Input: part model. Units: mm. Frame: model coordinates. Face numbers are marked on the shaded views. A direction names the side the tool comes from. Give positions to 0.01 mm unless a question says otherwise; leave off trailing zeros. Order: outer loops, then holes, each group sorted by start corner. A loop starts at its lowest first (then second) coordinate and runs counter-clockwise, first axis right, second up. Notation, with made-up numbers: M 17.25,6.5 L 57.25,6.5 A24 ccw 57.25,18.5 Z; hole C -9.75,64.5 d1. An arc over 180 degrees is marked long. Use a Markdown table: item, result.
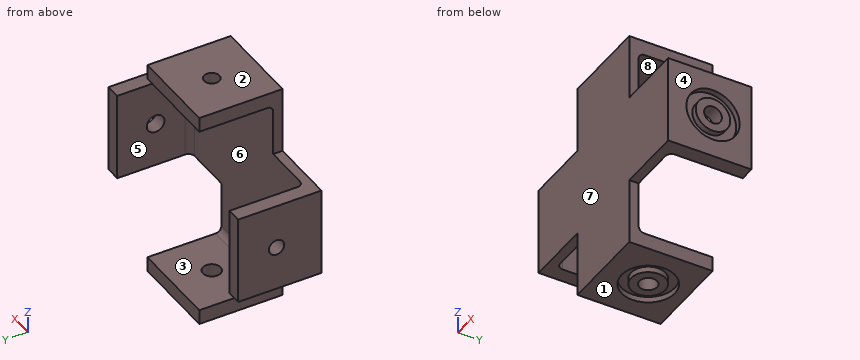
from build123d import *

# Parameters (mm, degrees)
BOSS_EXTRUDE1_DEPTH = 3.175
SKETCH4_W           = 5
SKETCH4_H           = 30
BOSS_EXTRUDE3_DEPTH = 25
FILLET1_R           = 2
SKETCH5_W           = 30
SKETCH5_H           = 5
BOSS_EXTRUDE4_DEPTH = 25
FILLET2_R           = 2
SKETCH6_R           = 2.6
CUT_EXTRUDE1_DEPTH  = 10
CIRPATTERN1_COUNT   = 2
CIRPATTERN1_ANGLE   = 90
SKETCH7_R           = 3
CUT_EXTRUDE2_DEPTH  = 10
CIRPATTERN2_COUNT   = 2
CIRPATTERN2_ANGLE   = 90
SKETCH10_R          = 9
SKETCH10_R_2        = 5.83
CUT_EXTRUDE9_DEPTH  = 2
CIRPATTERN4_COUNT   = 2
CIRPATTERN4_ANGLE   = 270


with BuildPart() as part:
    # Sketch1 → Boss-Extrude1 (new body)
    with BuildSketch(Plane(origin=(0, 0, 0), x_dir=(1, 0, 0), z_dir=(0, 1, 0))):
        Polygon((-15, 15), (-15, 37.5), (15, 37.5), (15, 15), (37.5, 15), (37.5, -15), (15, -15), (15, -37.5), (-15, -37.5), (-15, -15), (-37.5, -15), (-37.5, 15), align=None)
    extrude(amount=BOSS_EXTRUDE1_DEPTH)

    # Sketch4 → Boss-Extrude3 (add)
    with BuildSketch(Plane(origin=(0, 3.175, 0), x_dir=(1, 0, 0), z_dir=(0, 1, 0))):
        with Locations((-35, 0)):
            Rectangle(SKETCH4_W, SKETCH4_H)
        with Locations((35, 0)):
            Rectangle(SKETCH4_W, SKETCH4_H)
    extrude(amount=BOSS_EXTRUDE3_DEPTH)

    # Fillet1
    fillet1_edges = [part.edges().sort_by_distance(p)[0] for p in [
        (-32.5, 3.175, 0),
        (32.5, 3.175, 0),
    ]]
    fillet(fillet1_edges, radius=FILLET1_R)

    # Sketch5 → Boss-Extrude4 (add)
    with BuildSketch(Plane(origin=(0, 3.175, 0), x_dir=(1, 0, 0), z_dir=(0, 1, 0))):
        with Locations((0, -35)):
            Rectangle(SKETCH5_W, SKETCH5_H)
        with Locations((0, 35)):
            Rectangle(SKETCH5_W, SKETCH5_H)
    extrude(amount=BOSS_EXTRUDE4_DEPTH)

    # Fillet2
    fillet2_edges = [part.edges().sort_by_distance(p)[0] for p in [
        (0, 3.175, 32.5),
        (0, 3.175, -32.5),
    ]]
    fillet(fillet2_edges, radius=FILLET2_R)

    # Sketch6 → Cut-Extrude1 (cut)
    with BuildSketch(Plane.ZY.offset(37.5)):
        with Locations((0, 15.175)):
            Circle(SKETCH6_R)
    cut_extrude1 = extrude(amount=-CUT_EXTRUDE1_DEPTH, mode=Mode.SUBTRACT)

    # CirPattern1: Cut-Extrude1 ×2 about axis
    cirpattern1_axis = Axis((0, 3.175, 0), (0, 1, 0))
    for i in range(1, CIRPATTERN1_COUNT):
        add(cut_extrude1.rotate(cirpattern1_axis, i * CIRPATTERN1_ANGLE / (CIRPATTERN1_COUNT - 1)), mode=Mode.SUBTRACT)

    # Sketch7 → Cut-Extrude2 (cut)
    with BuildSketch(Plane(origin=(37.5, 0, 0), x_dir=(0, 0, -1), z_dir=(1, 0, 0))):
        with Locations((0, 15.175)):
            Circle(SKETCH7_R)
    cut_extrude2 = extrude(amount=-CUT_EXTRUDE2_DEPTH, mode=Mode.SUBTRACT)

    # CirPattern2: Cut-Extrude2 ×2 about axis
    cirpattern2_axis = Axis((0, 3.175, 0), (0, 1, 0))
    for i in range(1, CIRPATTERN2_COUNT):
        add(cut_extrude2.rotate(cirpattern2_axis, i * CIRPATTERN2_ANGLE / (CIRPATTERN2_COUNT - 1)), mode=Mode.SUBTRACT)

    # Sketch10 → Cut-Extrude9 (cut)
    with BuildSketch(Plane(origin=(0, 0, -37.5), x_dir=(-1, 0, 0), z_dir=(0, 0, -1))):
        with Locations((0, 15.175)):
            Circle(SKETCH10_R)
        with Locations((0, 15.175)):
            Circle(SKETCH10_R_2, mode=Mode.SUBTRACT)
    cut_extrude9 = extrude(amount=-CUT_EXTRUDE9_DEPTH, mode=Mode.SUBTRACT)

    # CirPattern4: Cut-Extrude9 ×2 about axis
    cirpattern4_axis = Axis((0, 3.175, 0), (0, 1, 0))
    for i in range(1, CIRPATTERN4_COUNT):
        add(cut_extrude9.rotate(cirpattern4_axis, i * CIRPATTERN4_ANGLE / (CIRPATTERN4_COUNT - 1)), mode=Mode.SUBTRACT)


solid = part.part
1) Reachability of the marked faces 4, 5, 6, 7 and 8 from +Z, -Z, +X, -X, +Y, -Y: full face, straight path, thin tool, end or side. Return the list, or none.
Response values:
| item | result |
|---|---|
| face 4 | +Z, -Z, +X, +Y, -Y |
| face 5 | +Z, -Z, +Y |
| face 6 | +Y |
| face 7 | +Z, -Z, +X, -X, -Y |
| face 8 | +X, -X, +Y |
2) Material intervals for line 1 (Y direction, x = 36.15, z = 0) (3 decimals); line 2 (X direction, y = 23, z = -10.5); line 3 (Y direction, x = 0, z = 33.65) (3 decimals), sorted ascending. Write a range as from..to.
Response values:
| item | result |
|---|---|
| line 1 | y = 0..6.175, 9.345..12.175, 18.175..21.005, 24.175..28.175 |
| line 2 | x = -37.5..-32.5, 32.5..37.5 |
| line 3 | y = 0..12.575, 17.775..28.175 |
3) Cut plane A-A on z = 0. Return loops of the section in (x, y) (3 decimals).
Response values:
| item | result |
|---|---|
| outline | M -37.5,0 L 37.5,0 L 37.5,6.175 L 35.5,6.175 L 35.5,9.345 L 37.5,9.345 L 37.5,12.175 L 32.5,12.175 L 32.5,5.175 A2 cw 30.5,3.175 L -30.5,3.175 A2 cw -32.5,5.175 L -32.5,12.575 L -37.5,12.575 Z; M -37.5,17.775 L -32.5,17.775 L -32.5,28.175 L -37.5,28.175 Z; M 32.5,18.175 L 37.5,18.175 L 37.5,21.005 L 35.5,21.005 L 35.5,24.175 L 37.5,24.175 L 37.5,28.175 L 32.5,28.175 Z |
4) Cut plane B-B on x = 0. Return loops of the section in (y, z) (3 decimals), and give its area (3 significant figures).
Response values:
| item | result |
|---|---|
| outline | M 0,-37.5 L 6.175,-37.5 L 6.175,-35.5 L 9.345,-35.5 L 9.345,-37.5 L 12.175,-37.5 L 12.175,-32.5 L 5.175,-32.5 A2 cw 3.175,-30.5 L 3.175,30.5 A2 cw 5.175,32.5 L 12.575,32.5 L 12.575,37.5 L 0,37.5 Z; M 17.775,32.5 L 28.175,32.5 L 28.175,37.5 L 17.775,37.5 Z; M 18.175,-37.5 L 21.005,-37.5 L 21.005,-35.5 L 24.175,-35.5 L 24.175,-37.5 L 28.175,-37.5 L 28.175,-32.5 L 18.175,-32.5 Z |
| area | 421 mm² |
5) First-contact query: pin 1 Ø7 at (x, y) = (24.5, 9.5) entering from +Z; pin 2 Ø5.5 at (x, y) = (1, 16) entering from -Z; pin 3 Ø12 at (x, z) = (-22, 20.5) entering from +Y (3 decimals); pin 4 Ø11 at (y, z) = (20.5, 28) entering from +X. Flat tips, straight axial feed; report the tip coordinate or a pass-through.
Response values:
| item | result |
|---|---|
| pin 1 | passes through |
| pin 2 | stops at z = -37.5 |
| pin 3 | stops at y = 3.175 |
| pin 4 | stops at x = 15 |
6) Cut plane C-C on y = 19.5. State how many separate pieces and enclosed holes the cut face has, and give its area (3 significant figures).
Response values:
| item | result |
|---|---|
| separate pieces | 4 |
| enclosed holes | 0 |
| area | 568 mm² |
7) Mould query, pull axis Z, two halves, no side actions, for the marked faces 1, 2 and 3. Classes: released by +Z, released by -Z, zero draft, split by the parting line, or undercut.
Response values:
| item | result |
|---|---|
| face 1 | released by -Z |
| face 2 | released by +Z |
| face 3 | undercut |
8) Cut plane D-D on z = 18.5. Return loops of the section in (x, y) (3 decimals), and give its area (4 significant figures).
Response values:
| item | result |
|---|---|
| outline | M -15,0 L 15,0 L 15,3.175 L -15,3.175 Z |
| area | 95.25 mm² |
